The listing builds one solid part. Answer for the finished solid, in the listing's coordinates (mm). A direction names the side the tool comes from. Coordinates: 2 decimals unless noted, no trailing zeros. Write each loop counter-clockwise with the first axis right and the second up, starting at its lowest first coordinate (ties: lowest second). Pieces come first, ordered by that corner, then holes. Notation, with made-up numbers: M 64.25,50 L 73.25,50 A20 cw 73.25,69 Z; hole C -27.75,61 d8. An arc over 180 degrees is marked long. Write item = value, one per line. Start each with the question number.
```python
from build123d import *

# Parameters (mm, degrees)
DRIVERDISKBASESKETCH_R   = 47.5
DRIVERDISKBASESKETCH_R_2 = 6.75
CENTERPAD_DEPTH          = 5
SKETCH_R                 = 47.5
SKETCH_R_2               = 25.25
OUTSIDEPAD_DEPTH         = 10
OBJ1          = 1.175
OBJ2_DEPTH         = 30
ROLLERSKETCH_R           = 4.7
ROLLERPAD_DEPTH          = 25
PINSKETCHFEMALESKETCH_R  = 1.425
PINJOINERPOCKET_DEPTH    = 15
PINPOLAR_COUNT           = 12


with BuildPart() as part:
    # DriverDiskBaseSketch → centerPad (new body)
    with BuildSketch(Plane.XY):
        Circle(DRIVERDISKBASESKETCH_R)
        Circle(DRIVERDISKBASESKETCH_R_2, mode=Mode.SUBTRACT)
    extrude(amount=CENTERPAD_DEPTH)

    # Sketch → outsidePad (join)
    with BuildSketch(Plane.XY):
        Circle(SKETCH_R)
        Circle(SKETCH_R_2, mode=Mode.SUBTRACT)
    extrude(amount=OUTSIDEPAD_DEPTH)

    with BuildSketch(Plane.XY):
        with Locations((-40.5, 0)):
            Circle(OBJ1)
    obj2 = extrude(amount=OBJ2_DEPTH)

    # rollerSketch → RollerPad (join)
    with BuildSketch(Plane.XY):
        with Locations((-40.5, 0)):
            Circle(ROLLERSKETCH_R)
    rollerpad = extrude(amount=ROLLERPAD_DEPTH)

    # pinSketchFemaleSketch → pinJoinerPocket (cut)
    with BuildSketch(Plane.XY):
        with Locations((-40.5, 0)):
            Circle(PINSKETCHFEMALESKETCH_R)
    pinjoinerpocket = extrude(amount=PINJOINERPOCKET_DEPTH, mode=Mode.SUBTRACT)

    # pinPolar: obj2, RollerPad, pinJoinerPocket ×12 about axis
    pinpolar_axis = Axis((0, 0, 0), (0, 0, 1))
    for i in range(1, PINPOLAR_COUNT):
        add(obj2.rotate(pinpolar_axis, i * 360 / PINPOLAR_COUNT))
        add(rollerpad.rotate(pinpolar_axis, i * 360 / PINPOLAR_COUNT))
        add(pinjoinerpocket.rotate(pinpolar_axis, i * 360 / PINPOLAR_COUNT), mode=Mode.SUBTRACT)


solid = part.part
```
1. For faces 1 (the face through (35, 20, 30)), 2 (the face through (-19.941, 36.465, 7.395)), 3 (the face through (0.207, 45.195, 17.395)), determine the directions among +Z, -Z, +X, -X, +Y, -Y from which every point of the face is accessible in a straight line to the end or side of a thin tool.
2. The part is cut by section D-D, the plane y = 28. Write down the section's boundary in (x, z).
3. The part is cut by section C-C, the plane x = -8. Write down the section's boundary in (y, z), and give its area (3 significant figures).
4. The part is cut by section A-A, the plane z = 19.25. Count the separate pieces of the cut face and the enclosed holes in it, and give its area (3 significant figures).
5. For a pull along Y with two mould halves and no side action, classify faces 4 (the face through (-31.111, -22.777, 17.395)), 5 (the face through (20, 35, 30)) as pulls with the +Y half, pulls with the -Y half, needs draft (parallel to the pull), parting line crosses it, or undercut.
6. Each of these flat-tipped pins is pushed along its axis until it touches: pin 1 (1 mm diameter, centred on x = -1.5, z = 8.5, fed in from +Y); pin 2 (12 mm diameter, centred on y = -19, z = 15.5, fed in from +X); pin 3 (1.5 mm diameter, centred on y = -33, z = 15.5, fed in from +X); pin 4 (7.5 mm diameter, centred on x = -22.5, y = 35, fed in from +Z). Where does it stop, or does it pass through?
7. Straight lines are drawn through the part: L1, parallel to X at y = 20.25, z = 10.75; L2, parallel to Y at x = 20.25, z = 7.75; L3, parallel to Z at x = -26.5, y = -39. For each, find the intervals that lie inside material, in ascending order. Write a range as [from, to].
Solution:
q1.face_1 = +Z, +X, -X, +Y, -Y
q1.face_2 = -Z
q1.face_3 = +Z
q2.outline = M -38.37,0 L 38.37,0 L 38.37,10 L -38.37,10 Z
q3.outline = M -46.82,0 L 46.82,0 L 46.82,10 L 23.95,10 L 23.95,5 L -23.95,5 L -23.95,10 L -46.82,10 Z
q3.area = 697 mm^2
q4.separate_pieces = 12
q4.enclosed_holes = 0
q4.area = 833 mm^2
q5.face_4 = undercut
q5.face_5 = needs draft
q6.pin_1 = 47.49
q6.pin_2 = 44.5
q6.pin_3 = 24.76
q6.pin_4 = 30
q7.L1 = [-39.77, -36.5], [-33.65, -30.37], [30.37, 33.65], [36.5, 39.77]
q7.L2 = [-42.97, -36.5], [-33.65, -15.08], [15.08, 33.65], [36.5, 42.97]
q7.L3 = [0, 10]
